Build history of the part. All positions in model axes, mm. A direction names the side the tool comes from. Round coordinates to 2 decimals unless told otherwise and drop trailing zeros. Loops run counter-clockwise (first coordinate to the right, second up) from the corner with the lowest first, then second, coordinate; pieces in that order, holes last.
Autodesk Inventor part; units mm, degrees
ref_plane "YZ Plane" through (0, 0, 0) normal (1, 0, 0) x (0, 1, 0)
ref_plane "XZ Plane" through (0, 0, 0) normal (0, 1, 0) x (-1, 0, 0)
ref_plane "XY Plane" through (0, 0, 0) normal (0, 0, 1) x (1, 0, 0)
sketch "Sketch1" plane through (0, 0, 0) normal (0, 0, 1) x (1, 0, 0)
  line L0 (0, 0) -> (0, 35)
  line L1 (0, 35) -> (20, 35)
  line L2 (20, 35) -> (20, 65)
  line L3 (20, 65) -> (0, 65)
  line L4 (0, 65) -> (0, 115.5325)
  line L5 (0, 115.5325) -> (90, 115.5325)
  line L6 (90, 115.5325) -> (278.4804, 25)
  line L7 (278.4804, 25) -> (278.4804, 0)
  line L8 (278.4804, 0) -> (0, 0)
  circle A0 centre (50, 25) radius 10
  dimension "d0" = 35
  dimension "d1" = 20
  dimension "d2" = 30
  dimension "d3" = 20
  dimension "d4" = 90
  dimension "d5" = 20
  dimension "d6" = 25
  dimension "d7" = 50
  dimension "d23" = 25
extrude "Extrusion1" add sketch "Sketch1" along normal blind 175
sketch "Sketch2" plane through (0, 115.5325, 0) normal (0, 1, 0) x (1, 0, 0)
  circle A0 centre (40, -25) radius 10
  line L0 (0, 0) -> (90, 0)
  line L1 (0, 0) -> (0, -175)
  dimension "d10" = 20
  dimension "d11" = 25
  dimension "d12" = 40
extrude "Extrusion2" cut sketch "Sketch2" against normal through all
sketch "Sketch3" plane through (0, 115.5325, 0) normal (0, 1, 0) x (1, 0, 0)
  line L0 (0, -50) -> (195.2781, -50)
  line L1 (0, 0) -> (90, 0)
  line L2 (0, 0) -> (0, -175)
  line L3 (0, -125) -> (195.2781, -125)
  line L4 (195.2781, -125) -> (195.2781, -50)
  line L5 (0, -125) -> (0, -50)
  dimension "d15" = 50
  dimension "d16" = 75
extrude "Extrusion3" cut sketch "Sketch3" against normal blind 25
sketch "Sketch4" plane through (0, 115.5325, 175) normal (0, 1, 0) x (1, 0, 0)
  line L0 (0, 0) -> (278.4804, 0)
  line L1 (75, 0) -> (320.0389, 141.4733)
  line L2 (320.0389, 141.4733) -> (320.0389, 0)
  line L3 (320.0389, 0) -> (75, 0)
  point P0 (0, 175)
  dimension "d19" = 75
  dimension "d20" = 30
extrude "Extrusion4" cut sketch "Sketch4" against normal through all
properties part number "HW 2 Part 3"
(1) Slice it at B-B on x = 110.5. List the corners of the cut face in (y, z), plus the area to 3 significant figures.
Responses:
outline: (0, 0) - (105.69, 0) - (105.69, 50) - (90.53, 50) - (90.53, 125) - (105.69, 125) - (105.69, 154.5) - (0, 154.5) - close
area: 15,200 mm2
(2) Pull direction X, two halves, no side cores. Call faces 1 (the face through (70, 90.532, 87)), 2 (the face through (59.54, 22, 86.28)), 3 (the face through (152.707, 45.738, 130.136)): +X half, -X half, draft (parallel to the pull), parting line (faces both ways), or undercut.
Responses:
face 1: draft
face 2: undercut
face 3: +X half
(3) Probe line 1 (Z direction, x = 27, y = 92); line 2 (Y direction, x = 50, z = 109); line 3 (Z direction, x = 40, y = 75). List the from-to ranges inside material, lowest first.
Responses:
line 1: z = 0 to 50, 125 to 175
line 2: y = 0 to 15, 35 to 90.53
line 3: z = 0 to 15, 35 to 175
(4) Slice it at A-A on z = 25. List the corners of the cut face in (x, y), plus the area to 3 significant figures.
Responses:
outline: (0, 0) - (30, 0) - (30, 115.53) - (0, 115.53) - (0, 65) - (20, 65) - (20, 35) - (0, 35) - close; (50, 0) - (278.48, 0) - (278.48, 25) - (90, 115.53) - (50, 115.53) - (50, 35) arc R10 cw to (50, 15) - close
area: 20,600 mm2
(5) Slice it at C-C on z = 91. List the corners of the cut face in (x, y).
Responses:
outline: (0, 0) - (220.49, 0) - (220.49, 52.85) - (142.05, 90.53) - (0, 90.53) - (0, 65) - (20, 65) - (20, 35) - (0, 35) - close; hole circle Ø20 at (50, 25)
(6) Slice it at D-D on x = 161. List the corners of the cut face in (y, z).
Responses:
outline: (0, 0) - (81.43, 0) - (81.43, 125.35) - (0, 125.35) - close
(7) Pin check, flat tips, straight feed: P1, Ø22.5, axis at x = 75.5, z = 70.5, coming from the +Y side; P2, Ø2, axis at x = 231.5, y = 31.5, coming from the +Z side; P3, Ø9, axis at y = 55, z = 79.5, coming from the -X side. Stop position of each tip, or through.
Responses:
P1: stops at y = 90.53
P2: stops at z = 85.22
P3: stops at x = 20
(8) Which spindle directions (+Z, -Z, +X, -X, +Y, -Y) get a long thin tool onto all of the face, cutting with end or side? Do faces 4 (the face through (30, 59, 25)), 5 (the face through (10, 35, 86)), 6 (the face through (54, 103, 125)). Say none if no direction does.
Responses:
face 4: +Y, -Y
face 5: +Z, -Z, -X
face 6: +X, -X, +Y
